Verification items for this drawing (mm, ordinates from the low corner). A direction names the side the tool comes from. Coordinates: 2 decimals unless noted, no trailing zeros. Loops run counter-clockwise (first coordinate to the right, second up) from the corner with the lowest first, then second, coordinate; pieces in that order, holes last.
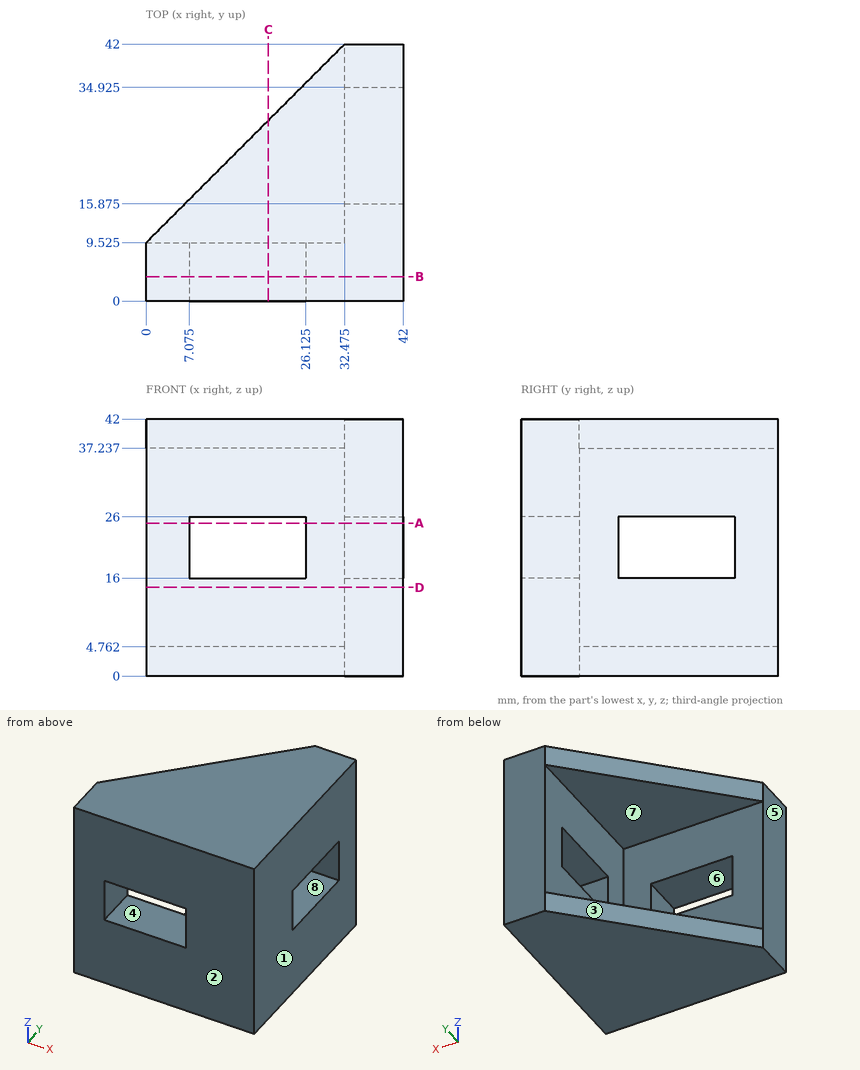
(1) Draft check along X on the marked faces 1, 2, 3 and 4. Enter one of: pulls with the +X half, pulls with the -X half, needs draft (parallel to the pull), parting line crosses it, or undercut.
(2) Section check C-C, the plane x = 20. Enter the section's corners in (y, z) (1 decimal).
(3) Set-up check for the marked faces 5, 6, 7 and 8: record each of +Z, -Z, +X, -X, +Y, -Y from which the full face is reachable in a straight line by a thin tool's end or side.
(4) Section check A-A, the plane z = 25. Enter the section's corners in (x, y) (1 decimal).
(5) Scan lines: line 1 along X through (y, z) = (5, 20.5) (1 decimal); line 2 along Y through (x, z) = (38, 20.5) (1 decimal); line 3 along Z through (x, y) = (23, 8.5). Record each from-to range of solid material in increasing order.
(6) Gauge pin test, flat ends, axial feed: P1, Ø12, axis at y = 32, z = 31, coming from the -X side (1 decimal); P2, Ø16, axis at x = 11.5, z = 23.5, coming from the +Y side (1 decimal). Record the tip position at first contact, or that the pin passes through.
(7) Section check B-B, the plane y = 4. Enter the section's corners in (x, z) (1 decimal), plus the area to 3 significant figures.
(8) Section check D-D, the plane z = 14.5. Enter the section's corners in (x, y) (1 decimal).
Determined:
1. face 1: pulls with the +X half
1. face 2: needs draft
1. face 3: pulls with the -X half
1. face 4: undercut
2. outline: (0, 0) - (29.5, 0) - (29.5, 4.8) - (9.5, 4.8) - (9.5, 16) - (0, 16) - close; (0, 26) - (9.5, 26) - (9.5, 37.2) - (29.5, 37.2) - (29.5, 42) - (0, 42) - close
3. face 5: +Z, -Z, -X, +Y, -Y
3. face 6: +Y, -Y
3. face 7: -X, +Y
3. face 8: +X, -X
4. outline: (0, 0) - (7.1, 0) - (7.1, 9.5) - (0, 9.5) - close; (26.1, 0) - (42, 0) - (42, 15.9) - (32.5, 15.9) - (32.5, 9.5) - (26.1, 9.5) - close; (32.5, 34.9) - (42, 34.9) - (42, 42) - (32.5, 42) - close
5. line 1: x = 0 to 7.1, 26.1 to 42
5. line 2: y = 0 to 15.9, 34.9 to 42
5. line 3: z = 0 to 16, 26 to 42
6. P1: stops at x = 32.5
6. P2: stops at y = 9.5
7. outline: (0, 0) - (42, 0) - (42, 42) - (0, 42) - close; hole (7.1, 16) - (26.1, 16) - (26.1, 26) - (7.1, 26) - close
7. area: 1,570 mm2
8. outline: (0, 0) - (42, 0) - (42, 42) - (32.5, 42) - (32.5, 9.5) - (0, 9.5) - close
